Build history of the part. All positions in model axes, mm. A direction names the side the tool comes from. Give positions to 0.01 mm unless a question says otherwise; leave off trailing zeros. Order: outer loops, then holes, each group sorted by start corner. A loop starts at its lowest first (then second) coordinate and runs counter-clockwise, first axis right, second up. Notation, with made-up numbers: (9.5, -16) -> (25.5, -16) arc R15 cw to (25.5, 9) -> close; hole circle Ø10 at (28, 57.5). An arc over 180 degrees is marked (long way). Write item = value, one per line. Start each with the question number.
from build123d import *

# Parameters (mm, degrees)
F0_W     = 6
F0_H     = 7.5
F0_H_2   = 7.7
F1_DEPTH = 10
F0_W_2   = 95
F0_H_3   = 10
F2_DEPTH = 10
F3_R     = 4.99999
F4_R     = 5


# Not quite as in the source:
# - a fillet or chamfer is up to 0.001 mm smaller than in the source, because OpenCascade refuses the exact size


with BuildPart() as f1:
    # F0 (on Top) → F1 (new body)
    with BuildSketch(Plane.XY):
        Polygon((-46.5609904528, 20.46333462), (-46.5609904528, 30.46333462), (-46.5609904528, 40.46333462), (-62.5609904528, 40.46333462), (-62.5609904528, 10.46333462), (-46.5609904528, 10.46333462), align=None)
        with Locations((-54.5609904528, 19.21333462)):
            Rectangle(F0_W, F0_H, mode=Mode.SUBTRACT)
        with Locations((-54.5609904528, 31.61333462)):
            Rectangle(F0_W, F0_H_2, mode=Mode.SUBTRACT)
    extrude(amount=F1_DEPTH)



with BuildPart() as f1b:
    # F0 (on Top) → F1, piece 2 (new body)
    with BuildSketch(Plane.XY):
        Polygon((48.4390095472, 40.46333462), (48.4390095472, 30.46333462), (48.4390095472, 20.46333462), (48.4390095472, 10.46333462), (64.4390095472, 10.46333462), (64.4390095472, 40.46333462), align=None)
        with Locations((56.4390095472, 19.21333462)):
            Rectangle(F0_W, F0_H, mode=Mode.SUBTRACT)
        with Locations((56.4390095472, 31.71333462)):
            Rectangle(F0_W, F0_H, mode=Mode.SUBTRACT)
    extrude(amount=F1_DEPTH)


with BuildPart() as f1_1:
    add(f1.part)

    add(f1b.part)  # F2 merges F1b
    # F0 (on Top) → F2 (join)
    with BuildSketch(Plane.XY):
        with Locations((0.9390095472, 25.46333462)):
            Rectangle(F0_W_2, F0_H_3)
    extrude(amount=F2_DEPTH)

    # F3 (radius 5 in the source; OpenCascade refuses exactly that, so slightly less here)
    f3_edges = [f1_1.edges().sort_by_distance(p)[0] for p in [
        (0.93901, 20.463335, 10),
        (0.93901, 30.463335, 10),
    ]]
    fillet(f3_edges, radius=F3_R)

    # F4
    f4_edges = [f1_1.edges().sort_by_distance(p)[0] for p in [
        (-62.56099, 10.463335, 5),
        (-46.56099, 10.463335, 5),
        (48.43901, 10.463335, 5),
        (64.43901, 10.463335, 5),
        (64.43901, 40.463335, 5),
        (48.43901, 40.463335, 5),
        (-46.56099, 40.463335, 5),
        (-62.56099, 40.463335, 5),
    ]]
    fillet(f4_edges, radius=F4_R)


solid = f1_1.part
(1) Cut at A-A, the plane y = 32.75. Give the cut face in (x, z).
(2) Wall check: line 1 (Y direction, x = -55, z = 8.25); line 2 (X direction, y = 29, z = 7.75); line 3 (X direction, y = 33.75, z = 2.25). Give the ranges that are in metal, low to high. Write a range as [from, to].
(3) Mould opens along X. For faces 1 (the face through (-62.561, 26, 5)), 2 (the face through (0, 20.463, 2)), 3 (the face through (1, 23, 0)) say: released by +X, released by -X, zero draft, split by the parting line, or undercut.
(4) 3-axis set-ups, long thin cutter, end or side, ignore diameter. For faces 4 (the face through (-46.561, 33, 5)), 5 (the face through (59.439, 19, 5)), 6 (the face through (-48.065, 11.889, 5.07)), 7 (the face through (0, 30.463, 2)): which of +Z, -Z, +X, -X, +Y, -Y reach the whole face in a straight line?
(5) Flat gauge pins, fed straight in: P1, Ø2, axis at x = 6.5, z = 8, coming from the -Y side; P2, Ø1, axis at x = 21, z = 8.5, coming from the -Y side; P3, Ø5, axis at x = 9.5, y = 19.5, coming from the +Z side. Where does each tip first touch, or does it go through?
(6) Cut at C-C, the plane z = 2. Give the number of separate pieces and of enclosed holes in the cut face, plus the area to 3 significant figures.
Results:
q1.outline = (-62.56, 0) -> (-57.56, 0) -> (-57.56, 10) -> (-62.56, 10) -> close; (-51.56, 0) -> (-46.56, 0) -> (-46.56, 10) -> (-51.56, 10) -> close; (48.44, 0) -> (53.44, 0) -> (53.44, 10) -> (48.44, 10) -> close; (59.44, 0) -> (64.44, 0) -> (64.44, 10) -> (59.44, 10) -> close
q2.line_1 = [10.46, 15.46], [22.96, 27.76], [35.46, 40.46]
q2.line_2 = [-62.56, -57.56], [-51.56, 53.44], [59.44, 64.44]
q2.line_3 = [-62.56, -57.56], [-51.56, -46.56], [48.44, 53.44], [59.44, 64.44]
q3.face_1 = released by -X
q3.face_2 = undercut
q3.face_3 = zero draft
q4.face_4 = +Z, +Y
q4.face_5 = +Z, -Z
q4.face_6 = +Z, -Z, -Y
q4.face_7 = +Z, -Z, +Y
q5.P1 = 20.88
q5.P2 = 21.46
q5.P3 = 8.61
q6.separate_pieces = 1
q6.enclosed_holes = 4
q6.area = 1,690 mm2
